```python
from build123d import *

# Parameters (mm, degrees)
SKETCH005_W  = 208
SKETCH005_H  = 40
SKETCH005_R  = 3.1
PAD005_DEPTH = 5
SKETCH006_W  = 208
SKETCH006_H  = 6
PAD006_DEPTH = 5
SKETCH007_W  = 41.5
SKETCH007_H  = 40
SKETCH007_R  = 3.2
PAD007_DEPTH = 5


with BuildPart() as part:
    # Sketch005 → Pad005 (new body)
    with BuildSketch(Plane.XY):
        with Locations((4, 0)):
            Rectangle(SKETCH005_W, SKETCH005_H)
        with Locations((8.1, -8.9)):
            Circle(SKETCH005_R, mode=Mode.SUBTRACT)
        with Locations((40.3, -8.9)):
            Circle(SKETCH005_R, mode=Mode.SUBTRACT)
        Polygon((93.75, 10), (90.875, 14.979646), (85.125, 14.979646), (82.25, 10), (85.125, 5.020354), (90.875, 5.020354), align=None, mode=Mode.SUBTRACT)
        Polygon((93.75, -10), (90.875, -5.020354), (85.125, -5.020354), (82.25, -10), (85.125, -14.979646), (90.875, -14.979646), align=None, mode=Mode.SUBTRACT)
        Polygon((-74.25, 10), (-77.125, 14.979646), (-82.875, 14.979646), (-85.75, 10), (-82.875, 5.020354), (-77.125, 5.020354), align=None, mode=Mode.SUBTRACT)
        Polygon((-74.25, -10), (-77.125, -5.020354), (-82.875, -5.020354), (-85.75, -10), (-82.875, -14.979646), (-77.125, -14.979646), align=None, mode=Mode.SUBTRACT)
        Polygon((-52.75, -10), (-55.625, -5.020354), (-61.375, -5.020354), (-64.25, -10), (-61.375, -14.979646), (-55.625, -14.979646), align=None, mode=Mode.SUBTRACT)
        Polygon((72.25, -10), (69.375, -5.020354), (63.625, -5.020354), (60.75, -10), (63.625, -14.979646), (69.375, -14.979646), align=None, mode=Mode.SUBTRACT)
    extrude(amount=PAD005_DEPTH)

    # Sketch006 (on Face43 of Pad005) → Pad006 (join)
    with BuildSketch(Plane(origin=(0, 0, 0), x_dir=(1, 0, 0), z_dir=(0, 0, -1))):
        with Locations((4, 0)):
            Rectangle(SKETCH006_W, SKETCH006_H)
    extrude(amount=PAD006_DEPTH)

    # Sketch007 (on Face6 of Pad006) → Pad007 (join)
    with BuildSketch(Plane(origin=(0, 0, 0), x_dir=(1, 0, 0), z_dir=(0, 0, -1))):
        with Locations((77.25, 0)):
            Rectangle(SKETCH007_W, SKETCH007_H)
        with Locations((88, 10)):
            Circle(SKETCH007_R, mode=Mode.SUBTRACT)
        with Locations((88, -10)):
            Circle(SKETCH007_R, mode=Mode.SUBTRACT)
        with Locations((66.5, 10)):
            Circle(SKETCH007_R, mode=Mode.SUBTRACT)
        with Locations((-69.25, 0)):
            Rectangle(SKETCH007_W, SKETCH007_H)
        with Locations((-58.5, 10)):
            Circle(SKETCH007_R, mode=Mode.SUBTRACT)
        with Locations((-80, -10)):
            Circle(SKETCH007_R, mode=Mode.SUBTRACT)
        with Locations((-80, 10)):
            Circle(SKETCH007_R, mode=Mode.SUBTRACT)
    extrude(amount=PAD007_DEPTH)


with BuildPart() as part_1:
    # Body007 placement: moved
    add(part.part.moved(Location((268, 278, 0))))


solid = part_1.part
```
The listing builds one solid part. Answer for the finished solid, in the listing's coordinates (mm). A direction names the side the tool comes from. Coordinates: 2 decimals unless noted, no trailing zeros. Loops run counter-clockwise (first coordinate to the right, second up) from the corner with the lowest first, then second, coordinate; pieces in that order, holes last. Notation, with made-up numbers: (70.5, 65) -> (90.5, 65) arc R30 ccw to (90.5, 87) -> close; hole circle Ø1 at (-21.5, 63.25). An arc over 180 degrees is marked (long way). Use one line per item in the form item = value. Start each with the question number.
Item 1: Flat-ended cylindrical pins translate along their axes: pin 1 Ø8 at (x, y) = (171.5, 266.5) entering from -Z; pin 2 Ø11 at (x, y) = (207, 265.5) entering from +Z; pin 3 Ø5.5 at (y, z) = (266, -3.5) entering from -X; pin 4 Ø5 at (x, y) = (356, 267) entering from +Z. Find the tip coordinate at first contact, or state that the pin passes through.
Item 2: The part is cut by section B-B on x = 209.5. Determine the outline of the cut face in (y, z), then the cut area to 3 significant figures.
Item 3: The part is cut by section D-D on x = 276.1. Determine the outline of the cut face in (y, z).
Item 4: Consider L1, parallel to X at y = 288, z = -1.15; L2, parallel to X at y = 268, z = -3.5; L3, parallel to Y at x = 188, z = -1.25. Determine where each line is inside the solid, lowest interval first. Write a range as [from, to].
Item 5: The part is cut by section C-C on x = 356. Determine the outline of the cut face in (y, z).
Item 6: A tool of negligible diameter and unlimited length cuts with its end or side. For faces 3 (the face through (360.292, 285.475, 2.465)), 4 (the face through (173, 290, 0)), 5 (the face through (271, 275, -2)), from which of +Z, -Z, +X, -X, +Y, -Y can it reach the whole face along a straight path? Write none if from no direction.
Item 7: The mould has two halves that part along X. Classify faces 1 (the face through (360.333, 290.455, 2.465)), 2 (the face through (173, 275, -2)): released by +X, released by -X, zero draft, split by the parting line, or undercut.
Item 8: The part is cut by section A-A on z = -3. Determine the outline of the cut face in (x, y).
Answer key:
q1.pin_1 = 0
q1.pin_2 = 5
q1.pin_3 = 178
q1.pin_4 = 0
q2.outline = (258, -5) -> (264.8, -5) -> (264.8, 0) -> (263.02, 0) -> (263.02, 5) -> (258, 5) -> close; (271.2, -5) -> (298, -5) -> (298, 5) -> (272.98, 5) -> (272.98, 0) -> (271.2, 0) -> close
q2.area = 318 mm2
q3.outline = (258, 0) -> (266, 0) -> (266, 5) -> (258, 5) -> close; (272.2, 0) -> (275, 0) -> (275, -5) -> (281, -5) -> (281, 0) -> (298, 0) -> (298, 5) -> (272.2, 5) -> close
q4.L1 = [178, 184.8], [191.2, 219.5], [324.5, 352.8], [359.2, 366]
q4.L2 = [178, 184.8], [191.2, 206.3], [212.7, 219.5], [324.5, 331.3], [337.7, 352.8], [359.2, 366]
q4.L3 = [258, 264.8], [271.2, 284.8], [291.2, 298]
q5.outline = (258, -5) -> (264.8, -5) -> (264.8, 0) -> (263.02, 0) -> (263.02, 5) -> (258, 5) -> close; (271.2, -5) -> (284.8, -5) -> (284.8, 0) -> (283.02, 0) -> (283.02, 5) -> (272.98, 5) -> (272.98, 0) -> (271.2, 0) -> close; (291.2, -5) -> (298, -5) -> (298, 5) -> (292.98, 5) -> (292.98, 0) -> (291.2, 0) -> close
q6.face_3 = +Z
q6.face_4 = -Z, -X, +Y
q6.face_5 = -Z, -Y
q7.face_1 = undercut
q7.face_2 = zero draft
q8.outline = (168, 275) -> (178, 275) -> (178, 258) -> (219.5, 258) -> (219.5, 275) -> (324.5, 275) -> (324.5, 258) -> (366, 258) -> (366, 275) -> (376, 275) -> (376, 281) -> (366, 281) -> (366, 298) -> (324.5, 298) -> (324.5, 281) -> (219.5, 281) -> (219.5, 298) -> (178, 298) -> (178, 281) -> (168, 281) -> close; hole circle Ø6.4 at (188, 268); hole circle Ø6.4 at (188, 288); hole circle Ø6.4 at (209.5, 268); hole circle Ø6.4 at (334.5, 268); hole circle Ø6.4 at (356, 268); hole circle Ø6.4 at (356, 288)
